from build123d import *

# Parameters (mm, degrees)
IZIM1_W                          = 90
IZIM1_H                          = 10
Y_KSEKLIK_EKSTR_ZYON1_DEPTH      = 20
IZIM6_W                          = 2
IZIM6_H                          = 1.5
KES_EKSTR_ZYON1_DEPTH            = 93.736184955
F_4_0MM_SAPLAMA_DELIKLERI3_D     = 5
F_4_0MM_SAPLAMA_DELIKLERI3_DEPTH = 8
IZIM14_R                         = 2
KES_EKSTR_ZYON2_DEPTH            = 93.736184955
IZIM13_R                         = 3.25
KES_EKSTR_ZYON4_DEPTH            = 6
KES_EKSTR_ZYON5_START            = -6
IZIM15_R                         = 3.25
KES_EKSTR_ZYON5_DEPTH            = 6


with BuildPart() as part:
    # Çizim1 → Yükseklik-Ekstrüzyon1 (new body)
    with BuildSketch(Plane.XY):
        with Locations((45, 5)):
            Rectangle(IZIM1_W, IZIM1_H)
    extrude(amount=Y_KSEKLIK_EKSTR_ZYON1_DEPTH)

    # Çizim6 → Kes-Ekstrüzyon1 (cut, through all)
    with BuildSketch(Plane.ZY):
        with Locations((5, 0.75)):
            Rectangle(IZIM6_W, IZIM6_H)
        with Locations((15, 0.75)):
            Rectangle(IZIM6_W, IZIM6_H)
    extrude(amount=-KES_EKSTR_ZYON1_DEPTH, mode=Mode.SUBTRACT)

    # Ø4.0mm Saplama Delikleri3
    with Locations(Plane(origin=(40, 10, 10), x_dir=(0, 0, 1), z_dir=(0, 1, 0))):
        with Locations((0, 0), (0, 40)):
            Hole(F_4_0MM_SAPLAMA_DELIKLERI3_D / 2, depth=F_4_0MM_SAPLAMA_DELIKLERI3_DEPTH)

    # Çizim14 → Kes-Ekstrüzyon2 (cut, through all)
    with BuildSketch(Plane.XY.offset(20)):
        with Locations((20, 5)):
            Circle(IZIM14_R)
        with Locations((70, 5)):
            Circle(IZIM14_R)
    extrude(amount=-KES_EKSTR_ZYON2_DEPTH, mode=Mode.SUBTRACT)

    # Çizim13 → Kes-Ekstrüzyon4 (cut)
    with BuildSketch(Plane.XY.offset(20)):
        with Locations((20, 5)):
            Circle(IZIM13_R)
        with Locations((70, 5)):
            Circle(IZIM13_R)
    extrude(amount=-KES_EKSTR_ZYON4_DEPTH, mode=Mode.SUBTRACT)

    # Çizim15 → Kes-Ekstrüzyon5 (cut)
    with BuildSketch(Plane(origin=(0, 0, 0), x_dir=(-1, 0, 0), z_dir=(0, 0, -1)).offset(KES_EKSTR_ZYON5_START)):
        with Locations(Location((-70, 5, 0), (0, 0, 180))):
            Circle(IZIM15_R)
        with Locations(Location((-20, 5, 0), (0, 0, 180))):
            Circle(IZIM15_R)
    extrude(amount=KES_EKSTR_ZYON5_DEPTH, mode=Mode.SUBTRACT)


solid = part.part
Can you work these out from the model? Positions are in its coordinate system, mm. A direction names the side the tool comes from. Give positions to 0.01 mm unless a question says otherwise; leave off trailing zeros. Order: outer loops, then holes, each group sorted by start corner. A loop starts at its lowest first (then second) coordinate and runs counter-clockwise, first axis right, second up. Notation, with made-up numbers: M 89,40 L 135,40 A20 cw 135,71 Z; hole C 72,-12 d11. An arc over 180 degrees is marked long. Use one line per item in the form item = value.
Item 1: If we section it at D-D, the plane x = 36: Write out the boundary of the cut face in (y, z), and give its area (3 significant figures).
Values follow:
outline = M 0,0 L 10,0 L 10,20 L 0,20 L 0,16 L 1.5,16 L 1.5,14 L 0,14 L 0,6 L 1.5,6 L 1.5,4 L 0,4 Z
area = 194 mm^2
Item 2: If we section it at C-C, the plane y = 6: Count the separate pieces of the cut face and the enclosed holes in it, and give its area (3 significant figures).
Values follow:
separate_pieces = 3
enclosed_holes = 2
area = 1,560 mm^2
Item 3: If we section it at A-A, the plane x = 20: Write out the boundary of the cut face in (y, z), and give its area (3 significant figures).
Values follow:
outline = M 0,0 L 1.75,0 L 1.75,6 L 3,6 L 3,14 L 1.75,14 L 1.75,20 L 0,20 L 0,16 L 1.5,16 L 1.5,14 L 0,14 L 0,6 L 1.5,6 L 1.5,4 L 0,4 Z; M 7,6 L 8.25,6 L 8.25,0 L 10,0 L 10,20 L 8.25,20 L 8.25,14 L 7,14 Z
area = 84.0 mm^2
Item 4: For faces 1 (the flat face through (21, 3, 14)), 2 (the flat face through (80, 2, 10)), 3 (the flat face through (72, 6, 6)), 4 (the flat face through (44, 1, 6)), which set-ups out of +Z, -Z, +X, -X, +Y, -Y let a thin tool reach every point of the face, with its end or its side?
Values follow:
face_1 = +Z
face_2 = +Y
face_3 = -Z
face_4 = +X, -X, -Y
Item 5: Thinking about a two-plate mould opening in Y: for faces 5 (the flat face through (40, 2, 10)), 6 (the flat face through (0, 5, 10)), 7 (the cylindrical face through (66.753, 4.857, 3.042)), 8 (the flat face through (21, 7, 6)), which applies, pulls with the +Y half, pulls with the -Y half, needs draft (parallel to the pull), parting line crosses it, or undercut?
Values follow:
face_5 = pulls with the +Y half
face_6 = needs draft
face_7 = undercut
face_8 = undercut
Item 6: If we section it at B-B, the plane z = 17: Write out the boundary of the cut face in (x, y).
Values follow:
outline = M 0,0 L 90,0 L 90,10 L 0,10 Z; hole C 20,5 d6.5; hole C 70,5 d6.5
Item 7: If I drill on line 1 along X through (y, z) = (5, 4.4); line 2 along Z through (x, y) = (27.5, 0.75); line 3 along X through (y, z) = (4, 11.75), over which ranges is the centre line in solid material (lowest first)? Write a range as [from, to].
Values follow:
line_1 = [0, 16.75], [23.25, 66.75], [73.25, 90]
line_2 = [0, 4], [6, 14], [16, 20]
line_3 = [0, 18.27], [21.73, 38.21], [41.79, 68.27], [71.73, 78.21], [81.79, 90]
Item 8: Will these pins go through, and if not, where does the flat tip stop? pin 1 Ø5 at (x, y) = (70, 5) entering from +Z; pin 2 Ø6 at (y, z) = (8.5, 6.5) entering from -X; pin 3 Ø1.6 at (x, z) = (46, 15) entering from -Y; pin 4 Ø6 at (x, y) = (20, 5) entering from -Z.
Values follow:
pin_1 = 14
pin_2 = 0
pin_3 = 1.5
pin_4 = 6
